```python
from build123d import *

# Parameters (mm, degrees)
F0_W      = 50
F0_H      = 40
F1_DEPTH  = 20
F2_W      = 48
F2_H      = 38
F3_DEPTH  = 19
F4_W      = 5
F4_H      = 5
F5_DEPTH  = 19
F6_R      = 1.5
F7_DEPTH  = 10
F9_R      = 2.5
F9_R_2    = 1.5
F10_DEPTH = 5


with BuildPart() as f1:
    # F0 (on Top) → F1 (new body)
    with BuildSketch(Plane.XY):
        with Locations((-39.054142, 36.971296)):
            Rectangle(F0_W, F0_H)
    extrude(amount=F1_DEPTH)

    # F2 (on face) → F3 (cut)
    with BuildSketch(Plane.XY.offset(20)):
        with Locations((-39.054142, 36.971296)):
            Rectangle(F2_W, F2_H)
    extrude(amount=-F3_DEPTH, mode=Mode.SUBTRACT)

    # F4 (on face) → F5 (join)
    with BuildSketch(Plane.XY.offset(1)):
        with Locations((-60.554142, 53.471296)):
            Rectangle(F4_W, F4_H)
        with Locations((-60.554142, 20.471296)):
            Rectangle(F4_W, F4_H)
        with Locations((-17.554142, 53.471296)):
            Rectangle(F4_W, F4_H)
        with Locations((-17.554142, 20.471296)):
            Rectangle(F4_W, F4_H)
    extrude(amount=F5_DEPTH)

    # F6 (on face) → F7 (cut)
    with BuildSketch(Plane.XY.offset(20)):
        with Locations((-60.554142, 53.471296)):
            Circle(F6_R)
        with Locations((-60.554142, 20.471296)):
            Circle(F6_R)
        with Locations((-17.554142, 20.471296)):
            Circle(F6_R)
        with Locations((-17.554142, 53.471296)):
            Circle(F6_R)
    extrude(amount=-F7_DEPTH, mode=Mode.SUBTRACT)

    # F9 (on face) → F10 (join)
    with BuildSketch(Plane.XY.offset(1)):
        with Locations((-43.054142, 32.971296)):
            Circle(F9_R)
        with Locations((-43.054142, 32.971296)):
            Circle(F9_R_2, mode=Mode.SUBTRACT)
        with Locations((-28.054142, 42.971296)):
            Circle(F9_R)
        with Locations((-28.054142, 42.971296)):
            Circle(F9_R_2, mode=Mode.SUBTRACT)
    extrude(amount=F10_DEPTH)


solid = f1.part
```
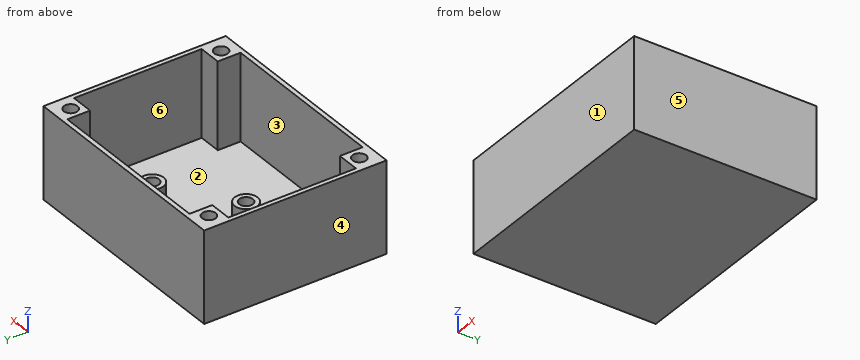
Read the model definition and answer for the solid it produces. Units are mm, in the model's axes. Face numbers are marked on the shaded views. A direction names the side the tool comes from. Give positions to 0.01 mm unless a question says otherwise; leave off trailing zeros. Order: outer loops, then holes, each group sorted by start corner. A loop starts at its lowest first (then second) coordinate and runs counter-clockwise, first axis right, second up.
(1) For the marked faces 5 and 6, determine the directions among +Z, -Z, +X, -X, +Y, -Y from which every point of the face is accessible in a straight line to the end or side of a thin tool.
(2) For a pull along Y with two mould halves and no side action, classify the marked faces 1, 2, 3 and 4 as released by +Y, released by -Y, zero draft, split by the parting line, or undercut.
(3) Given pin 1 (2 mm diameter, centred on x = -35, y = 34, fed in from +Z); pin 2 (1.5 mm diameter, centred on x = -17.5, y = 21, fed in from +Z); pin 3 (3.5 mm diameter, centred on x = -28, y = 43, fed in from +Z), each flat-ended and moving along its own axis, determine where each tip first touches the part or whether it passes through.
(4) Find section B-B (x = -22). Give the vertices of the cut face in (y, z), plus the area to 3 significant figures.
(5) Find section D-D (z = 15.5). Give the vertices of the cut face in (x, y).
(6) Find section A-A (z = 4). Give the vertices of the cut face in (x, y).
(7) Find section C-C (y = 47.5). Give the vertices of the cut face in (x, z).
(8) Straight lines are drawn through the part: L1, parallel to Y at x = -60.5, z = 10.5; L2, parallel to Y at x = -57, z = 8.5; L3, parallel to X at y = 38.5, z = 17.25. For each, find the intervals that lie inside material, in ascending order.
Result sheet:
1. face 5: +Z, -Z, +X, +Y, -Y
1. face 6: +Z
2. face 1: released by -Y
2. face 2: undercut
2. face 3: undercut
2. face 4: zero draft
3. pin 1: stops at z = 1
3. pin 2: stops at z = 10
3. pin 3: stops at z = 6
4. outline: (16.97, 0) - (56.97, 0) - (56.97, 20) - (55.97, 20) - (55.97, 1) - (17.97, 1) - (17.97, 20) - (16.97, 20) - close
4. area: 78.0 mm2
5. outline: (-64.05, 16.97) - (-14.05, 16.97) - (-14.05, 56.97) - (-64.05, 56.97) - close; hole (-63.05, 22.97) - (-58.05, 22.97) - (-58.05, 17.97) - (-20.05, 17.97) - (-20.05, 22.97) - (-15.05, 22.97) - (-15.05, 50.97) - (-20.05, 50.97) - (-20.05, 55.97) - (-58.05, 55.97) - (-58.05, 50.97) - (-63.05, 50.97) - close; hole circle Ø3 at (-60.55, 20.47); hole circle Ø3 at (-60.55, 53.47); hole circle Ø3 at (-17.55, 20.47); hole circle Ø3 at (-17.55, 53.47)
6. outline: (-64.05, 16.97) - (-14.05, 16.97) - (-14.05, 56.97) - (-64.05, 56.97) - close; circle Ø5 at (-43.05, 32.97); circle Ø5 at (-28.05, 42.97); hole (-63.05, 22.97) - (-58.05, 22.97) - (-58.05, 17.97) - (-20.05, 17.97) - (-20.05, 22.97) - (-15.05, 22.97) - (-15.05, 50.97) - (-20.05, 50.97) - (-20.05, 55.97) - (-58.05, 55.97) - (-58.05, 50.97) - (-63.05, 50.97) - close; hole circle Ø3 at (-43.05, 32.97); hole circle Ø3 at (-28.05, 42.97)
7. outline: (-64.05, 0) - (-14.05, 0) - (-14.05, 20) - (-15.05, 20) - (-15.05, 1) - (-63.05, 1) - (-63.05, 20) - (-64.05, 20) - close
8. L1: y = 16.97 to 18.97, 21.97 to 22.97, 50.97 to 51.97, 54.97 to 56.97
8. L2: y = 16.97 to 17.97, 55.97 to 56.97
8. L3: x = -64.05 to -63.05, -15.05 to -14.05
